For this review, take the finished solid that the model builds, in its own axes (mm). Face numbers are marked on the shaded views. A direction names the side the tool comes from. Give positions to 0.01 mm unless a question says otherwise; leave off trailing zeros. Order: outer loops, then holes, each group sorted by start corner. A loop starts at its lowest first (then second) coordinate and runs counter-clockwise, first axis right, second up. Notation, with made-up numbers: (26, 22) - (67, 22) arc R13 cw to (67, 42) - close; hole circle Ø9 at (78, 54). An arc over 180 degrees is marked (long way). One line per item, written item: value.
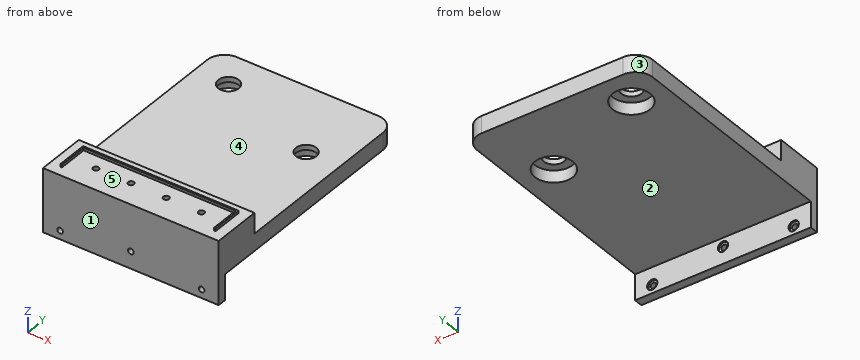
```python
from build123d import *

# Parameters (mm, degrees)
SKETCH2_R           = 11.05
BOSS_EXTRUDE2_DEPTH = 10
BOSS_EXTRUDE3_START = 7
SKETCH2_4_R         = 11.05
SKETCH2_4_R_2       = 6
BOSS_EXTRUDE3_DEPTH = 3
SKETCH3_W           = 102.73844499
SKETCH3_H           = 28.8
BOSS_EXTRUDE4_DEPTH = 12
SKETCH4_W           = 5.8
SKETCH4_H           = 17.75
CUT_EXTRUDE2_DEPTH  = 8
SKETCH4_7_W         = 5.8
SKETCH4_7_H         = 17.75
SKETCH4_7_R         = 1.7
BOSS_EXTRUDE5_DEPTH = 5.3
BOSS_EXTRUDE6_DEPTH = 1.5
SKETCH6_W           = 102.73844499
SKETCH6_H           = 25
BOSS_EXTRUDE7_DEPTH = 5
SKETCH7_R           = 1.65
CUT_EXTRUDE3_DEPTH  = 5
SKETCH7_6_R         = 3
SKETCH7_6_R_2       = 1.65
CUT_EXTRUDE4_DEPTH  = 1


with BuildPart() as part:
    # Sketch2 → Boss-Extrude2 (new body)
    with BuildSketch(Plane.XY):
        with BuildLine():
            Line((-10, 0), (-92.73844499, 0))
            ThreePointArc((-92.73844499, 0), (-99.809512802, -2.928932188), (-102.73844499, -10))
            Line((-102.73844499, -10), (-102.73844499, -142.20223365))
            Line((-102.73844499, -142.20223365), (0, -142.20223365))
            Line((0, -142.20223365), (0, -10))
            ThreePointArc((0, -10), (-2.928932188, -2.928932188), (-10, 0))
        make_face()
        with Locations((-82.73844499, -20.4)):
            Circle(SKETCH2_R, mode=Mode.SUBTRACT)
        with Locations((-20, -44.29848365)):
            Circle(SKETCH2_R, mode=Mode.SUBTRACT)
    extrude(amount=BOSS_EXTRUDE2_DEPTH)

    # Sketch2_4 → Boss-Extrude3 (add)
    # profile 1 of 2: a face of its own
    with BuildSketch(Plane.XY.offset(BOSS_EXTRUDE3_START)):
        with Locations((-82.73844499, -20.4)):
            Circle(SKETCH2_4_R)
        with Locations((-82.73844499, -20.4)):
            Circle(SKETCH2_4_R_2, mode=Mode.SUBTRACT)
    # profile 2 of 2: a face of its own
    with BuildSketch(Plane.XY.offset(BOSS_EXTRUDE3_START)):
        with Locations((-20, -44.29848365)):
            Circle(SKETCH2_4_R)
        with Locations((-20, -44.29848365)):
            Circle(SKETCH2_4_R_2, mode=Mode.SUBTRACT)
    extrude(amount=BOSS_EXTRUDE3_DEPTH)

    # Sketch3 → Boss-Extrude4 (add)
    with BuildSketch(Plane.XY.offset(10)):
        with Locations((-51.369222495, -127.80223365)):
            Rectangle(SKETCH3_W, SKETCH3_H)
    extrude(amount=BOSS_EXTRUDE4_DEPTH)

    # Sketch4 → Cut-Extrude2 (cut)
    with BuildSketch(Plane.XY.offset(22)):
        with Locations((-61.64306899, -122.27723365)):
            Rectangle(SKETCH4_W, SKETCH4_H)
        with Locations((-82.19075699, -122.27723365)):
            Rectangle(SKETCH4_W, SKETCH4_H)
        with Locations((-41.09538099, -122.27723365)):
            Rectangle(SKETCH4_W, SKETCH4_H)
        with Locations((-20.54769299, -122.27723365)):
            Rectangle(SKETCH4_W, SKETCH4_H)
    extrude(amount=-CUT_EXTRUDE2_DEPTH, mode=Mode.SUBTRACT)

    # Sketch4_7 → Boss-Extrude5 (add)
    # profile 1 of 4: a face of its own
    with BuildSketch(Plane.XY.offset(22)):
        with Locations((-61.64306899, -122.27723365)):
            Rectangle(SKETCH4_7_W, SKETCH4_7_H)
        with Locations((-61.64306899, -127.85223365)):
            Circle(SKETCH4_7_R, mode=Mode.SUBTRACT)
    # profile 2 of 4: a face of its own
    with BuildSketch(Plane.XY.offset(22)):
        with Locations((-82.19075699, -122.27723365)):
            Rectangle(SKETCH4_7_W, SKETCH4_7_H)
        with Locations((-82.19075699, -127.85223365)):
            Circle(SKETCH4_7_R, mode=Mode.SUBTRACT)
    # profile 3 of 4: a face of its own
    with BuildSketch(Plane.XY.offset(22)):
        with Locations((-41.09538099, -122.27723365)):
            Rectangle(SKETCH4_7_W, SKETCH4_7_H)
        with Locations((-41.09538099, -127.85223365)):
            Circle(SKETCH4_7_R, mode=Mode.SUBTRACT)
    # profile 4 of 4: a face of its own
    with BuildSketch(Plane.XY.offset(22)):
        with Locations((-20.54769299, -122.27723365)):
            Rectangle(SKETCH4_7_W, SKETCH4_7_H)
        with Locations((-20.54769299, -127.85223365)):
            Circle(SKETCH4_7_R, mode=Mode.SUBTRACT)
    extrude(amount=-BOSS_EXTRUDE5_DEPTH)

    # Sketch5 → Boss-Extrude6 (add)
    with BuildSketch(Plane.XY.offset(22)):
        Polygon((-95.78844499, -136.50223365), (-96.78844499, -136.50223365), (-96.78844499, -118.10223365), (-5.95, -118.10223365), (-5.95, -136.50223365), (-6.95, -136.50223365), (-6.95, -119.10223365), (-95.78844499, -119.10223365), align=None)
    extrude(amount=BOSS_EXTRUDE6_DEPTH)

    # Sketch6 → Boss-Extrude7 (add)
    with BuildSketch(Plane.XZ.offset(142.20223365)):
        with Locations((-51.369222495, -2.5)):
            Rectangle(SKETCH6_W, SKETCH6_H)
    extrude(amount=-BOSS_EXTRUDE7_DEPTH)

    # Sketch7 → Cut-Extrude3 (cut)
    with BuildSketch(Plane(origin=(-101.64020113, -137.20223365, -23.052849439), x_dir=(-1, 0, 0), z_dir=(0, 1, 0))):
        with Locations(Location((-91.64020113, 13.052849439, 0), (0, 0, 90))):
            Circle(SKETCH7_R)
        with Locations(Location((-50.270978635, 18.052849439, 0), (0, 0, 90))):
            Circle(SKETCH7_R)
        with Locations(Location((-8.90175614, 13.052849439, 0), (0, 0, 90))):
            Circle(SKETCH7_R)
    extrude(amount=-CUT_EXTRUDE3_DEPTH, mode=Mode.SUBTRACT)

    # Sketch7_6 → Cut-Extrude4 (cut)
    # profile 1 of 3: a face of its own
    with BuildSketch(Plane(origin=(-101.64020113, -137.20223365, -23.052849439), x_dir=(-1, 0, 0), z_dir=(0, 1, 0))):
        with Locations(Location((-91.64020113, 13.052849439, 0), (0, 0, 90))):
            Circle(SKETCH7_6_R)
        with Locations(Location((-91.64020113, 13.052849439, 0), (0, 0, 90))):
            Circle(SKETCH7_6_R_2, mode=Mode.SUBTRACT)
    # profile 2 of 3: a face of its own
    with BuildSketch(Plane(origin=(-101.64020113, -137.20223365, -23.052849439), x_dir=(-1, 0, 0), z_dir=(0, 1, 0))):
        with Locations(Location((-50.270978635, 18.052849439, 0), (0, 0, 90))):
            Circle(SKETCH7_6_R)
        with Locations(Location((-50.270978635, 18.052849439, 0), (0, 0, 90))):
            Circle(SKETCH7_6_R_2, mode=Mode.SUBTRACT)
    # profile 3 of 3: a face of its own
    with BuildSketch(Plane(origin=(-101.64020113, -137.20223365, -23.052849439), x_dir=(-1, 0, 0), z_dir=(0, 1, 0))):
        with Locations(Location((-8.90175614, 13.052849439, 0), (0, 0, 90))):
            Circle(SKETCH7_6_R)
        with Locations(Location((-8.90175614, 13.052849439, 0), (0, 0, 90))):
            Circle(SKETCH7_6_R_2, mode=Mode.SUBTRACT)
    extrude(amount=-CUT_EXTRUDE4_DEPTH, mode=Mode.SUBTRACT)


solid = part.part
```
(1) Draft analysis for pull direction X (two halves, no side actions). For the marked faces 3, 4 and 5, state which applies: pulls with the +X half, pulls with the -X half, needs draft (parallel to the pull), parting line crosses it, or undercut.
Answers below:
face 3: pulls with the -X half
face 4: needs draft
face 5: undercut
(2) Take a section at B-B (y = -20.4). Write out the cut boundary in (x, z).
Answers below:
outline: (-102.74, 0) - (-93.79, 0) - (-93.79, 7) - (-88.74, 7) - (-88.74, 10) - (-102.74, 10) - close; (-76.74, 7) - (-71.69, 7) - (-71.69, 0) - (0, 0) - (0, 10) - (-76.74, 10) - close
(3) Take a section at C-C (z = 8.5). Write out the cut boundary in (x, y).
Answers below:
outline: (-102.74, -142.2) - (0, -142.2) - (0, -10) arc R10 ccw to (-10, 0) - (-92.74, 0) arc R10 ccw to (-102.74, -10) - close; hole circle Ø12 at (-82.74, -20.4); hole circle Ø12 at (-20, -44.3)
(4) Machinability: for the marked faces 1 and 2, which of the approach directions +Z, -Z, +X, -X, +Y, -Y give a long, thin tool a straight path to every point of the face, cutting with its end or side? Answer none if there is none.
Answers below:
face 1: +Z, -Z, +X, -X, -Y
face 2: -Z, +X, -X, +Y
(5) Wall thickness on line 1 (X direction, y = -141.15, z = -10); line 2 (X direction, y = -139.55, z = -5); line 3 (Z direction, x = -44, y = -105): over which ranges is each line inside the solid? List them lowest first. Write a range as from..to.
Answers below:
line 1: x = -102.74..-94.39, -91.09..-11.65, -8.35..0
line 2: x = -102.74..-53.02, -49.72..0
line 3: z = 0..10
(6) For P1, Ø6.5, axis at x = -80.5, y = -25.5, coming from the -Z side; P2, Ø1.3, axis at x = -19.5, z = 15.5, coming from the +Y side; P3, Ø4.5, axis at x = -82.19, y = -127.85, coming from the +Z side, all flat-tipped, find the tip position at first contact; note any pin that passes through.
Answers below:
P1: stops at z = 7
P2: stops at y = -131.15
P3: stops at z = 22
(7) Take a section at D-D (y = -86). Write out the cut boundary in (x, z).
Answers below:
outline: (-102.74, 0) - (0, 0) - (0, 10) - (-102.74, 10) - close
(8) Take a section at A-A (z = -5). Write out the cut boundary in (x, y).
Answers below:
outline: (-102.74, -142.2) - (-53.02, -142.2) - (-53.02, -138.2) - (-54.37, -138.2) - (-54.37, -137.2) - (-102.74, -137.2) - close; (-49.72, -142.2) - (0, -142.2) - (0, -137.2) - (-48.37, -137.2) - (-48.37, -138.2) - (-49.72, -138.2) - close
